Autodesk Inventor part; units mm, degrees
ref_plane "YZ Plane" through (0, 0, 0) normal (1, 0, 0) x (0, 1, 0)
ref_plane "XZ Plane" through (0, 0, 0) normal (0, 1, 0) x (-1, 0, 0)
ref_plane "XY Plane" through (0, 0, 0) normal (0, 0, 1) x (1, 0, 0)
sketch "Sketch1" plane through (0, 0, 0) normal (0, 0, 1) x (1, 0, 0)
  circle A0 centre (0, 0) radius 3.75
  line L0 (1.25, -6.25) -> (-1.25, -6.25)
  line L1 (-1.25, -6.25) -> (-1.25, 6.25) construction
  line L2 (-1.25, 6.25) -> (1.25, 6.25)
  line L3 (1.25, 6.25) -> (1.25, -6.25) construction
  circle A1 centre (0, 0) radius 5.25
  line L4 (1.25, -5.099) -> (1.25, -6.25)
  line L5 (-1.25, -6.25) -> (-1.25, -5.099)
  line L6 (-1.25, 6.25) -> (-1.25, 5.099)
  line L7 (1.25, 6.25) -> (1.25, 5.099)
  arc A2 (-1.25, -5.099) -> (1.25, -5.099) centre (0, 0) ccw
  arc A3 (1.25, 5.099) -> (-1.25, 5.099) centre (0, 0) ccw
  point P0 (0, 6.25)
  point P1 (1.25, 0)
  dimension "d1" = 7.5
  dimension "d10" = 2.5
  dimension "d11" = 12.5
  dimension "d12" = 10.5
extrude "Extrusion1" add sketch "Sketch1" along normal blind 12
sketch "Sketch5" plane through (0, 0, 0) normal (0, 0, -1) x (-1, 0, 0)
  circle A0 centre (0, 0) radius 3.75
  circle A1 centre (0, 0) radius 3.75
  line L0 (-1.25, -6.25) -> (-1.25, -5.099)
  line L1 (1.25, -6.25) -> (-1.25, -6.25)
  line L2 (1.25, -5.099) -> (1.25, -6.25)
  arc A2 (1.25, -5.099) -> (1.25, 5.099) centre (0, 0) ccw
  line L3 (1.25, 6.25) -> (1.25, 5.099)
  line L4 (-1.25, 6.25) -> (1.25, 6.25)
  line L5 (-1.25, 5.099) -> (-1.25, 6.25)
  arc A3 (-1.25, 5.099) -> (-1.25, -5.099) centre (0, 0) ccw
  circle A4 centre (0, 0) radius 1.5
  dimension "d13" = 3
extrude "Extrusion4" add sketch "Sketch5" along normal blind 2 contours A0 | L0 A3 L5 L4 L3 A2 L2 L1
sketch "Sketch6" plane through (0, 0, 0) normal (0, 0, 1) x (1, 0, 0)
  line L0 (0.625, 6.25) -> (-0.625, 6.25)
  line L1 (-0.625, 6.25) -> (-0.625, -6.25) construction
  line L2 (-0.625, -6.25) -> (0.625, -6.25)
  line L3 (0.625, -6.25) -> (0.625, 6.25) construction
  line L4 (-1.25, 6.25) -> (1.25, 6.25)
  circle A0 centre (0, 0) radius 1.5 construction
  arc A1 (0.625, 1.3636) -> (-0.625, 1.3636) centre (0, 0) ccw
  arc A2 (-0.625, -1.3636) -> (0.625, -1.3636) centre (0, 0) ccw
  line L5 (0.625, 6.25) -> (0.625, 1.3636)
  line L6 (-0.625, 6.25) -> (-0.625, 1.3636)
  line L7 (0.625, -1.3636) -> (0.625, -6.25)
  line L8 (-0.625, -1.3636) -> (-0.625, -6.25)
  point P0 (0, 0)
  point P1 (0, 6.25)
  point P2 (0.625, 0)
  dimension "d16" = 1.25
extrude "Extrusion5" add sketch "Sketch6" along normal blind 2
sketch "Sketch9" plane through (0, 0, 12) normal (0, 0, 1) x (1, 0, 0)
  circle A0 centre (0, 0) radius 3.75 construction
  line L0 (1.25, -6.25) -> (1.25, -5.099)
  arc A1 (1.25, -5.099) -> (1.25, 5.099) centre (0, 0) ccw
  line L1 (1.25, 5.099) -> (1.25, 6.25)
  line L2 (1.25, 6.25) -> (-1.25, 6.25)
  line L3 (-1.25, 6.25) -> (-1.25, 5.099)
  arc A2 (-1.25, 5.099) -> (-1.25, -5.099) centre (0, 0) ccw
  line L4 (-1.25, -5.099) -> (-1.25, -6.25)
  line L5 (-1.25, -6.25) -> (1.25, -6.25)
  circle A3 centre (0, 0) radius 4.75
  dimension "d23" = 9.5
extrude "Extrusion7" add sketch "Sketch9" along normal blind 4
properties part number "AA042" material "ABS Plastic"
The model under review builds one solid part; all positions refer to its coordinate system, in mm. A direction names the side the tool comes from. Round coordinates to 2 decimals unless told otherwise and drop trailing zeros. Loops run counter-clockwise (first coordinate to the right, second up) from the corner with the lowest first, then second, coordinate; pieces in that order, holes last.
1) Tool access review of faces 5 (the face through (2, 0, 0)), 6 (the face through (-1.25, -6, 7)), 7 (the face through (1.25, 6, 7)), 8 (the face through (-1.25, 6, 7)): name each direction out of +Z, -Z, +X, -X, +Y, -Y from which nothing blocks a thin tool from reaching the whole face with its end or side.
Values follow:
face 5: +Z
face 6: +Z, -Z, -X, -Y
face 7: +Z, -Z, +X, +Y
face 8: +Z, -Z, -X, +Y
2) Consider section C-C on y = 0. State the section outline as (x, z) points, then the cut area to 3 significant figures.
Values follow:
outline: (-5.25, -2) - (-1.5, -2) - (-1.5, 0) - (-3.75, 0) - (-3.75, 12) - (-4.75, 12) - (-4.75, 16) - (-5.25, 16) - (-5.25, 12) - close; (1.5, -2) - (5.25, -2) - (5.25, 0) - (5.25, 16) - (4.75, 16) - (4.75, 12) - (3.75, 12) - (3.75, 0) - (1.5, 0) - close
area: 55.0 mm2
3) Consider section D-D on x = 3.25. State the section outline as (y, z) points, then the cut area to 3 significant figures.
Values follow:
outline: (-4.12, -2) - (4.12, -2) - (4.12, 0) - (4.12, 16) - (3.46, 16) - (3.46, 12) - (1.87, 12) - (1.87, 0) - (-1.87, 0) - (-1.87, 12) - (-3.46, 12) - (-3.46, 16) - (-4.12, 16) - (-4.12, 0) - close
area: 75.8 mm2
4) The part is to be moulded in two halves that separate along Y. For faces 1 (the face through (-5.25, 0.1, -0.99)), 2 (the face through (0, -1.5, 1)), 3 (the face through (-5, 1, 16)), 4 (the face through (-2, 0, 0)), say which applies: pulls with the +Y half, pulls with the -Y half, needs draft (parallel to the pull), parting line crosses it, or undercut.
Values follow:
face 1: parting line crosses it
face 2: undercut
face 3: needs draft
face 4: undercut
5) Wall thickness on line 1 along X through (y, z) = (0, 2.75); line 2 along X through (y, z) = (0, -0.6); line 3 along Y through (x, z) = (0, 10.25): over which ranges is each line inside the solid? List them lowest first.
Values follow:
line 1: x = -5.25 to -3.75, 3.75 to 5.25
line 2: x = -5.25 to -1.5, 1.5 to 5.25
line 3: y = -6.25 to -3.75, 3.75 to 6.25
6) Consider section A-A on x = 0. State the section outline as (y, z) points.
Values follow:
outline: (-6.25, -2) - (-1.5, -2) - (-1.5, 2) - (-3.75, 2) - (-3.75, 12) - (-4.75, 12) - (-4.75, 16) - (-6.25, 16) - close; (1.5, -2) - (6.25, -2) - (6.25, 16) - (4.75, 16) - (4.75, 12) - (3.75, 12) - (3.75, 2) - (1.5, 2) - close
7) Consider section B-B on z = 0.25. State the section outline as (x, y) points (3 decimals).
Values follow:
outline: (-1.25, -6.25) - (1.25, -6.25) - (1.25, -5.099) arc R5.25 ccw to (1.25, 5.099) - (1.25, 6.25) - (-1.25, 6.25) - (-1.25, 5.099) arc R5.25 ccw to (-1.25, -5.099) - close; hole (-0.625, -3.698) - (-0.625, -1.364) arc R1.5 ccw to (0.625, -1.364) - (0.625, -3.698) arc R3.75 ccw to (0.625, 3.698) - (0.625, 1.364) arc R1.5 ccw to (-0.625, 1.364) - (-0.625, 3.698) arc R3.75 ccw to start
8) Clearance check with flat-ended pins moving along their axes: P1, Ø1, axis at y = 3, z = 0.5, coming from the -X side; P2, Ø3, axis at x = -4, z = 6.5, coming from the +Y side; P3, Ø1, axis at y = 2, z = 0.5, coming from the +X side. State where each tip first meets the part, or that it passes through.
Values follow:
P1: stops at x = -4.62
P2: stops at y = 4.62
P3: stops at x = 5.03
